Autodesk Inventor part; units mm, degrees
ref_plane "YZ Plane" through (0, 0, 0) normal (1, 0, 0) x (0, 1, 0)
ref_plane "XZ Plane" through (0, 0, 0) normal (0, 1, 0) x (-1, 0, 0)
ref_plane "XY Plane" through (0, 0, 0) normal (0, 0, 1) x (1, 0, 0)
sketch "Sketch1" plane through (0, 0, 0) normal (1, 0, 0) x (0, 1, 0)
  line L0 (-6, -4) -> (6, -4)
  line L1 (6, -4) -> (6, 4)
  line L2 (6, 4) -> (-6, 4)
  line L3 (-6, 4) -> (-6, -4)
  line L4 (-6, -4) -> (6, 4) construction
  line L5 (6, -4) -> (-6, 4) construction
  point P0 (0, 0)
  dimension "d0" = 12
  dimension "d1" = 8
extrude "Extrusion1" add sketch "Sketch1" along normal blind 25
sketch "Sketch2" plane through (0, -6, -4) normal (0, -1, 0) x (1, 0, 0)
  line L0 (0, 8) -> (25, 8)
  line L1 (0, 8) -> (0, 0)
  point P0 (0, 4)
  point P1 (12.5, 4)
  point P2 (12.5, 8)
  point P3 (0, 4)
hole "Hole1" at (12.5, -6, 0) direction (0, 1, 0) diameter 5 depth 3 tip angle 118
chamfer "Chamfer1" distance 1 angle 45 2 edges at (12.5, 6, -4) (12.5, 6, 4)
properties part number "Jaw" material "Aluminum 6061"
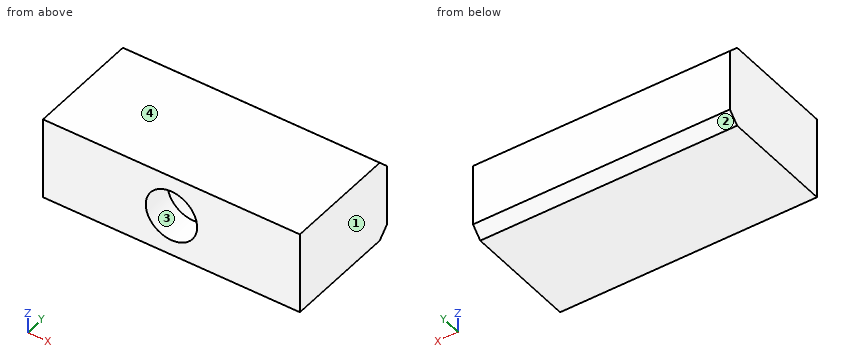
Input: part model. Units: mm. Frame: model coordinates. Face numbers are marked on the shaded views. Round coordinates to 2 decimals unless told otherwise and drop trailing zeros. Order: outer loops, then holes, each group sorted by start corner. A loop starts at its lowest first (then second) coordinate and runs counter-clockwise, first axis right, second up.
1. Pin query (flat end, axial travel): P1, Ø1, axis at y = 3, z = 1.5, coming from the -X side. Return the tip coordinate at first contact, or that it passes through.
The answers:
P1: stops at x = 0
2. Material intervals for line 1 (X direction, y = -5, z = 0); line 2 (Z direction, x = 12.5, y = -4.3); line 3 (X direction, y = -2.5, z = 0.75), sorted ascending.
The answers:
line 1: x = 0 to 10, 15 to 25
line 2: z = -4 to -2.5, 2.5 to 4
line 3: x = 0 to 11.01, 13.99 to 25
3. Mould query, pull axis Z, two halves, no side actions, for the marked faces 1, 2, 3 and 4. Classes: released by +Z, released by -Z, zero draft, split by the parting line, or undercut.
The answers:
face 1: zero draft
face 2: released by -Z
face 3: undercut
face 4: released by +Z
4. Cut plane A-A, the plane y = -5.25. Output: boundary loops of the cut face in (x, z).
The answers:
outline: (0, -4) - (25, -4) - (25, 4) - (0, 4) - close; hole circle Ø5 at (12.5, 0)
